```python
from build123d import *

# Parameters (mm, degrees)
PAD_DEPTH = 4


with BuildPart() as part:
    # Sketch → Pad (new body)
    with BuildSketch(Plane.XY):
        with BuildLine():
            ThreePointArc((0, 10), (-10, 0), (0, -10))
            Line((0, -10), (121.237625, -10))
            ThreePointArc((121.237625, -10), (131.237625, 0), (121.237625, 10))
            Line((0, 10), (121.237625, 10))
        make_face()
        with BuildLine():
            ThreePointArc((0, 3), (-3, 0), (0, -3))
            Line((0, -3), (50, -3))
            ThreePointArc((50, -3), (53, 0), (50, 3))
            Line((0, 3), (50, 3))
        make_face(mode=Mode.SUBTRACT)
        with BuildLine():
            ThreePointArc((70, 3), (67, 0), (70, -3))
            Line((70, -3), (120, -3))
            ThreePointArc((120, -3), (123, 0), (120, 3))
            Line((70, 3), (120, 3))
        make_face(mode=Mode.SUBTRACT)
    extrude(amount=PAD_DEPTH)


solid = part.part
```
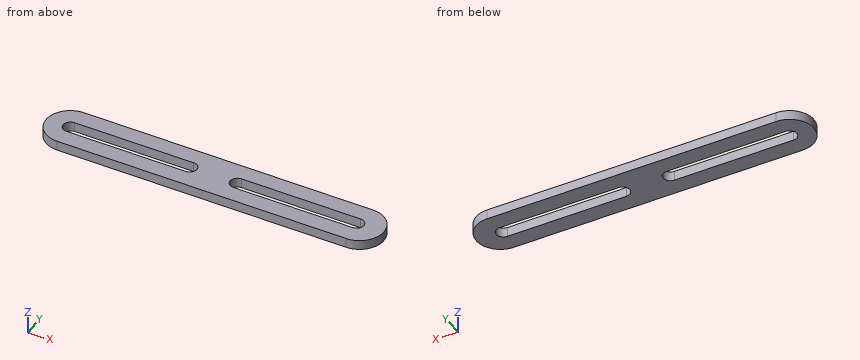
Geometry: final body of the model. Coordinates: model frame, mm. Round coordinates to 2 decimals unless told otherwise and drop trailing zeros. Loops run counter-clockwise (first coordinate to the right, second up) from the corner with the lowest first, then second, coordinate; pieces in that order, holes last.
Item 1: Section C-C, the plane z = 1.95. Output: boundary loops of the cut face in (x, y), plus the area to 3 significant figures.
Checked values:
outline: (0, -10) - (121.24, -10) arc R10 ccw to (121.24, 10) - (0, 10) arc R10 ccw to start; hole (0, -3) - (50, -3) arc R3 ccw to (50, 3) - (0, 3) arc R3 ccw to start; hole (70, -3) - (120, -3) arc R3 ccw to (120, 3) - (70, 3) arc R3 ccw to start
area: 2,080 mm2
Item 2: Section B-B, the plane x = 76. Output: boundary loops of the cut face in (y, z), plus the area to 3 significant figures.
Checked values:
outline: (-10, 0) - (-3, 0) - (-3, 4) - (-10, 4) - close; (3, 0) - (10, 0) - (10, 4) - (3, 4) - close
area: 56.0 mm2
Item 3: Section A-A, the plane y = 0. Output: boundary loops of the cut face in (x, z), plus the area to 3 significant figures.
Checked values:
outline: (-10, 0) - (-3, 0) - (-3, 4) - (-10, 4) - close; (53, 0) - (67, 0) - (67, 4) - (53, 4) - close; (123, 0) - (131.24, 0) - (131.24, 4) - (123, 4) - close
area: 117 mm2
Item 4: Line query: L1, parallel to Y at x = 7.5, z = 1.7; L2, parallel to X at y = 0.5, z = 0.65; L3, parallel to X at y = 2, z = 1. Output: solid intervals per line, ascending.
Checked values:
L1: y = -10 to -3, 3 to 10
L2: x = -9.99 to -2.96, 52.96 to 67.04, 122.96 to 131.23
L3: x = -9.8 to -2.24, 52.24 to 67.76, 122.24 to 131.04
Item 5: Contact query for flat-ended pins moving along their axis: P1, Ø6, axis at x = 82.5, y = -5, coming from the -Z side; P2, Ø2, axis at x = 86, y = 1.5, coming from the +Z side. Output: stop coordinate, or through.
Checked values:
P1: stops at z = 0
P2: passes through
Item 6: Section D-D, the plane y = -8.5. Output: boundary loops of the cut face in (x, z), plus the area to 3 significant figures.
Checked values:
outline: (-5.27, 0) - (126.51, 0) - (126.51, 4) - (-5.27, 4) - close
area: 527 mm2
